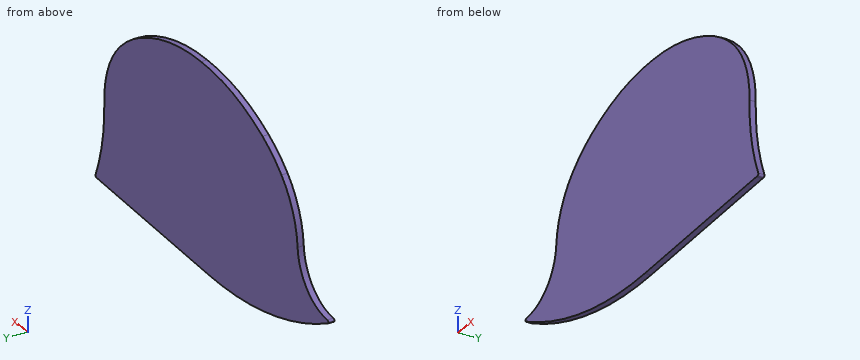
```python
from build123d import *

# Parameters (mm, degrees)
BOSS_EXTRUDE1_DEPTH = 3


with BuildPart() as part:
    # Sketch1 → Boss-Extrude1 (new body)
    with BuildSketch(Plane(origin=(0, 0, 0), x_dir=(1, 0, 0), z_dir=(0, 1, 0))):
        with BuildLine():
            Line((125.334448741, 60.70559707), (34.689006477, 64.197109776))
            ThreePointArc((34.689006477, 64.197109776), (-15.13644212, 59.561512619), (-62.05150383, 42.153437665))
            ThreePointArc((-62.05150383, 42.153437665), (-62.647956965, 41.28649391), (-61.869388221, 40.578554275))
            ThreePointArc((-61.869388221, 40.578554275), (-45.258927275, 33.746363612), (-37.601267241, 17.499933699))
            ThreePointArc((-37.601267241, 17.499933699), (-33.623817753, 2.15297615), (-24.412676642, -10.750670229))
            ThreePointArc((-24.412676642, -10.750670229), (-17.089531788, -16.87593356), (-8.972231882, -21.901542344))
            ThreePointArc((-8.972231882, -21.901542344), (15.331470951, -31.037864787), (41.132426556, -33.945277559))
            ThreePointArc((41.132426556, -33.945277559), (66.933382162, -31.037864787), (91.237084995, -21.901542344))
            ThreePointArc((91.237084995, -21.901542344), (99.354384901, -16.87593356), (106.677529755, -10.750670229))
            ThreePointArc((106.677529755, -10.750670229), (116.726166056, 4.084607563), (119.930653965, 21.713896145))
            ThreePointArc((119.930653965, 21.713896145), (121.458201516, 41.048643152), (127.049993776, 59.620064816))
            ThreePointArc((127.049993776, 59.620064816), (126.959504732, 60.402154552), (126.242784377, 60.727983579))
            ThreePointArc((126.242784377, 60.727983579), (125.788970047, 60.70244749), (125.334448741, 60.70559707))
        make_face()
    extrude(amount=BOSS_EXTRUDE1_DEPTH)


solid = part.part
```
Build history of the part. All positions in model axes, mm. Give positions to 0.01 mm unless a question says otherwise; leave off trailing zeros. Order: outer loops, then holes, each group sorted by start corner. A loop starts at its lowest first (then second) coordinate and runs counter-clockwise, first axis right, second up. Notation, with made-up numbers: M -27.5,81.5 L -18.5,81.5 A27 ccw -18.5,99.5 Z; hole C 83,54.25 d3. An arc over 180 degrees is marked long. Return JSON: item names as keys, results as strings.
Q1. Band-saw the part on B-B (x = 22). Give the cut face in (y, z), then the cut area to 3 significant figures.
Answer list:
{"outline": "M 0,-64.26 L 3,-64.26 L 3,32.41 L 0,32.41 Z", "area": "290 mm^2"}
Q2. Flat gauge pin, fed straight in: pin 1 (1.5 mm diameter, centred on x = 82.5, y = 0.5, fed in from +Z). Where does the tip first touch, or does it go through?
Answer list:
{"pin 1": "stops at z = 26.29"}
Q3. Band-saw the part on C-C (z = -38). Give the cut face in (x, y).
Answer list:
{"outline": "M -51.34,0 L 120.94,0 L 120.94,3 L -51.34,3 Z"}
Q4. Band-saw the part on A-A (y = 1.85). Give the cut face in (x, z).
Answer list:
{"outline": "M -62.05,-42.15 A191.15 ccw 34.69,-64.2 L 125.33,-60.71 A7.2 cw 126.24,-60.73 A0.8 ccw 127.05,-59.62 A90.96 cw 119.93,-21.71 A43.43 ccw 106.68,10.75 A67.2 ccw 91.24,21.9 A105.23 ccw 41.13,33.95 A105.23 ccw -8.97,21.9 A67.2 ccw -24.41,10.75 A43.52 ccw -37.6,-17.5 A24.83 cw -61.87,-40.58 A0.8 ccw Z"}
Q5. Wall check: probe 1 along X at (y, z) = (1.4, -18); probe 2 along X at (y, z) = (1.9, -6); probe 3 along Z at (x, y) = (-43.5, 2.7). Give the ranges that are in metal, low to high. Write a range as from..to.
Answer list:
{"probe 1": "x = -37.64..119.88", "probe 2": "x = -35.2..117.46", "probe 3": "z = -50.73..-31.89"}
